For this review, take the finished solid that the model builds, in its own axes (mm). Face numbers are marked on the shaded views. Round coordinates to 2 decimals unless told otherwise and drop trailing zeros. Write each loop counter-clockwise with the first axis right and the second up, starting at its lowest first coordinate (ties: lowest second). Pieces come first, ordered by that corner, then holes.
from build123d import *

# Parameters (mm, degrees)
CROQUIS1_W              = 20
CROQUIS1_H              = 25
SALIENTE_EXTRUIR4_DEPTH = 16
CORTAR_EXTRUIR1_START   = 10
CROQUIS4_W              = 21
CROQUIS4_H              = 12
CORTAR_EXTRUIR1_DEPTH   = 18
SALIENTE_EXTRUIR6_START = -10
CROQUIS5_W              = 21
CROQUIS5_H              = 1
SALIENTE_EXTRUIR6_DEPTH = 24
SALIENTE_EXTRUIR7_START = 10
CROQUIS7_W              = 2
CROQUIS7_H              = 8
SALIENTE_EXTRUIR7_DEPTH = 4
SALIENTE_EXTRUIR8_START = 16
CROQUIS8_W              = 12.75
CROQUIS8_H              = 11
SALIENTE_EXTRUIR8_DEPTH = 3
CROQUIS9_W              = 9.75
CROQUIS9_H              = 1.5
CORTAR_EXTRUIR2_DEPTH   = 11.5
CROQUIS11_W             = 6
CROQUIS11_H             = 4.75
CORTAR_EXTRUIR4_DEPTH   = 16.5
CROQUIS12_W             = 6
CROQUIS12_H             = 4.75
CORTAR_EXTRUIR5_DEPTH   = 33


with BuildPart() as part:
    # Croquis1 → Saliente-Extruir4 (new body)
    with BuildSketch(Plane(origin=(0, 0, 0), x_dir=(1, 0, 0), z_dir=(0, 1, 0))):
        Rectangle(CROQUIS1_W, CROQUIS1_H)
    extrude(amount=SALIENTE_EXTRUIR4_DEPTH)

    # Croquis4 → Cortar-Extruir1 (cut)
    with BuildSketch(Plane(origin=(0, 0, 0), x_dir=(0, 0, -1), z_dir=(1, 0, 0)).offset(CORTAR_EXTRUIR1_START)):
        with Locations((0, 8)):
            Rectangle(CROQUIS4_W, CROQUIS4_H)
    extrude(amount=-CORTAR_EXTRUIR1_DEPTH, mode=Mode.SUBTRACT)

    # Croquis5 → Saliente-Extruir6 (add)
    with BuildSketch(Plane(origin=(0, 0, 0), x_dir=(0, 0, -1), z_dir=(1, 0, 0)).offset(SALIENTE_EXTRUIR6_START)):
        with Locations((0, 8)):
            Rectangle(CROQUIS5_W, CROQUIS5_H)
    extrude(amount=SALIENTE_EXTRUIR6_DEPTH)

    # Croquis7 → Saliente-Extruir7 (add)
    with BuildSketch(Plane(origin=(0, 0, 0), x_dir=(0, 0, -1), z_dir=(1, 0, 0)).offset(SALIENTE_EXTRUIR7_START)):
        with Locations((-11.5, 8)):
            Rectangle(CROQUIS7_W, CROQUIS7_H)
        with Locations((11.5, 8)):
            Rectangle(CROQUIS7_W, CROQUIS7_H)
    extrude(amount=SALIENTE_EXTRUIR7_DEPTH)

    # Croquis8 → Saliente-Extruir8 (add)
    with BuildSketch(Plane(origin=(0, 0, 0), x_dir=(1, 0, 0), z_dir=(0, 1, 0)).offset(SALIENTE_EXTRUIR8_START)):
        with Locations((-3.625, 0)):
            Rectangle(CROQUIS8_W, CROQUIS8_H)
    extrude(amount=SALIENTE_EXTRUIR8_DEPTH)

    # Croquis9 → Cortar-Extruir2 (cut, symmetric)
    with BuildSketch(Plane.XY):
        with Locations((-3.625, 16.75)):
            Rectangle(CROQUIS9_W, CROQUIS9_H)
    extrude(amount=CORTAR_EXTRUIR2_DEPTH, both=True, mode=Mode.SUBTRACT)

    # Croquis11 → Cortar-Extruir4 (cut, symmetric)
    with BuildSketch(Plane.XY):
        with Locations((2, 10.875)):
            Rectangle(CROQUIS11_W, CROQUIS11_H)
    extrude(amount=CORTAR_EXTRUIR4_DEPTH, both=True, mode=Mode.SUBTRACT)

    # Croquis12 → Cortar-Extruir5 (cut)
    with BuildSketch(Plane(origin=(0, 0, 0), x_dir=(0, 0, -1), z_dir=(1, 0, 0))):
        with Locations((0, 4.375)):
            Rectangle(CROQUIS12_W, CROQUIS12_H)
    extrude(amount=-CORTAR_EXTRUIR5_DEPTH, mode=Mode.SUBTRACT)


solid = part.part
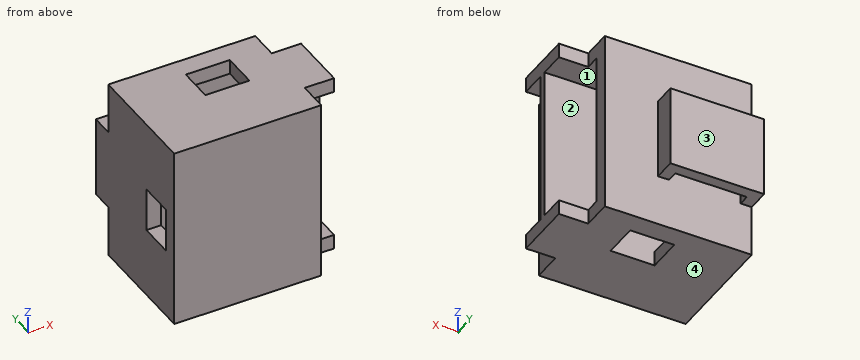
(1) We need section B-B, the plane y = 4.5. Give the boundary of the cut face in (x, z), and give its area (3 significant figures).
Geometry check:
outline: (-10, -12.5) - (14, -12.5) - (14, -10.5) - (-8, -10.5) - (-8, -3) - (-10, -3) - close; (-10, 3) - (-8, 3) - (-8, 10.5) - (14, 10.5) - (14, 12.5) - (-10, 12.5) - close
area: 126 mm2
(2) We need section D-D, the plane x = 3.25. Give the boundary of the cut face in (y, z).
Geometry check:
outline: (0, -12.5) - (8.5, -12.5) - (8.5, 12.5) - (0, 12.5) - close; (13.25, -12.5) - (16, -12.5) - (16, 12.5) - (13.25, 12.5) - (13.25, 10.5) - (14, 10.5) - (14, -10.5) - (13.25, -10.5) - close; hole (2, -10.5) - (7.5, -10.5) - (7.5, 10.5) - (2, 10.5) - close
(3) We need section A-A, the plane x = -6.5. Give the boundary of the cut face in (y, z).
Geometry check:
outline: (0, -12.5) - (16, -12.5) - (16, 12.5) - (0, 12.5) - close; (17.5, -5.5) - (19, -5.5) - (19, 5.5) - (17.5, 5.5) - close; hole (2, -10.5) - (7.5, -10.5) - (7.5, 10.5) - (2, 10.5) - close; hole (8.5, -10.5) - (14, -10.5) - (14, 10.5) - (8.5, 10.5) - close
(4) For line 1 along Y through (x, z) = (-4.5, -3.25); line 2 along Y through (x, z) = (6.5, 6); line 3 along X through (y, z) = (17.25, 0.5), list the stretches that pass through material, from the lowest coordinate up.
Geometry check:
line 1: y = 0 to 2, 7.5 to 8.5, 14 to 16, 17.5 to 19
line 2: y = 0 to 2, 7.5 to 8.5, 14 to 16
line 3: x = -10 to -8.5, 1.25 to 2.75
(5) We need section C-C, the plane z = 4.5. Give the boundary of the cut face in (x, y), and give its area (3 significant figures).
Geometry check:
outline: (-10, 0) - (10, 0) - (10, 2) - (-8, 2) - (-8, 7.5) - (14, 7.5) - (14, 8.5) - (-8, 8.5) - (-8, 14) - (10, 14) - (10, 16) - (2.75, 16) - (2.75, 19) - (-10, 19) - close; hole (-8.5, 16) - (1.25, 16) - (1.25, 17.5) - (-8.5, 17.5) - close
area: 150 mm2
(6) Mouldability with a two-part tool opening along Z and no side actions: class the marked faces 1, 2, 3 and 4 as pulls with the +Z half, pulls with the -Z half, needs draft (parallel to the pull), parting line crosses it, or undercut.
Geometry check:
face 1: undercut
face 2: undercut
face 3: needs draft
face 4: pulls with the -Z half
(7) For pin 1 Ø2 at (x, z) = (12, 11.5) entering from +Y; pin 2 Ø3 at (y, z) = (11.5, 2.5) entering from +X; pin 3 Ø1 at (y, z) = (17, 0) entering from +X, all flat-tipped, find the tip position at first contact; note any pin that passes through.
Geometry check:
pin 1: stops at y = 12
pin 2: stops at x = -8
pin 3: stops at x = 2.75
